For this review, take the finished solid that the model builds, in its own axes (mm). A direction names the side the tool comes from. Give positions to 0.01 mm unless a question says otherwise; leave off trailing zeros. Write each loop counter-clockwise with the first axis right and the second up, starting at its lowest first coordinate (ties: lowest second). Pieces come first, ordered by that corner, then holes. Notation, with made-up numbers: (57, -35) -> (106, -35) arc R21 cw to (106, -27) -> close; hole circle Ø2 at (41, -11.75). An arc over 180 degrees is marked (long way). Write item = value, one per line.
```python
from build123d import *

# Parameters (mm, degrees)
SKETCH1_R           = 28.4
BOSS_EXTRUDE1_DEPTH = 7
SKETCH2_R           = 28.4
BOSS_EXTRUDE3_DEPTH = 7
SKETCH4_R           = 7.5
BOSS_EXTRUDE4_DEPTH = 11
CUT_EXTRUDE1_DEPTH  = 10


with BuildPart() as part:
    # Sketch1 → Boss-Extrude1 (new body)
    with BuildSketch(Plane.XY):
        Circle(SKETCH1_R)
    extrude(amount=BOSS_EXTRUDE1_DEPTH)

    # Sketch2 → Boss-Extrude3 (add)
    with BuildSketch(Plane.XY.offset(7)):
        with Locations((1.88, 0)):
            Circle(SKETCH2_R)
    extrude(amount=BOSS_EXTRUDE3_DEPTH)

    # Sketch4 → Boss-Extrude4 (add)
    with BuildSketch(Plane.XY.offset(14)):
        with Locations((0.94, 0)):
            Circle(SKETCH4_R)
    extrude(amount=BOSS_EXTRUDE4_DEPTH)

    # Sketch6 → Cut-Extrude1 (cut)
    with BuildSketch(Plane.XY.offset(25)):
        with BuildLine():
            Line((0.44, 2.770056), (1.44, 2.770056))
            Line((1.44, 2.770056), (1.44, 4.472135955))
            ThreePointArc((1.44, 4.472135955), (0.94, -4.5), (0.44, 4.472135955))
            Line((0.44, 4.472135955), (0.44, 2.770056))
        make_face()
    extrude(amount=-CUT_EXTRUDE1_DEPTH, mode=Mode.SUBTRACT)


solid = part.part
```
(1) Tool access review of faces 1 (the face through (0.44, 4, 20)), 2 (the face through (-27, 2, 7)), 3 (the face through (29, 0, 7)): name each direction out of +Z, -Z, +X, -X, +Y, -Y from which nothing blocks a thin tool from reaching the whole face with its end or side.
Answers below:
face_1 = +Z
face_2 = +Z, -X
face_3 = -Z, +X
(2) Take a section at B-B (y = 0). Write out the cut boundary in (x, z).
Answers below:
outline = (-28.4, 0) -> (28.4, 0) -> (28.4, 7) -> (30.28, 7) -> (30.28, 14) -> (8.44, 14) -> (8.44, 25) -> (5.44, 25) -> (5.44, 15) -> (-3.56, 15) -> (-3.56, 25) -> (-6.56, 25) -> (-6.56, 14) -> (-26.52, 14) -> (-26.52, 7) -> (-28.4, 7) -> close
(3) To check wall thickness, follow probe 1 along Y at (x, z) = (0.94, 17); probe 2 along Z at (x, y) = (-17.5, -21); probe 3 along Z at (x, y) = (15, 20). State the ranges of each line that lie inside material, in increasing order.
Answers below:
probe_1 = -7.5 to -4.5, 2.77 to 7.5
probe_2 = 0 to 7
probe_3 = 0 to 14
(4) Take a section at D-D (z = 9.25). Write out the cut boundary in (x, y), plus the area to 3 significant figures.
Answers below:
outline = circle Ø56.8 at (1.88, 0)
area = 2,530 mm^2
(5) Take a section at A-A (z = 18). Write out the cut boundary in (x, y).
Answers below:
outline = circle Ø15 at (0.94, 0); hole (0.44, 2.77) -> (0.44, 4.47) arc R4.5 ccw (long way) to (1.44, 4.47) -> (1.44, 2.77) -> close
(6) For pin 1 (6 mm diameter, centred on x = -7.5, y = 9.5, fed in from +Z); pin 2 (1.4 mm diameter, centred on y = 4, z = 18, fed in from +X) (3 decimals); pin 3 (3 mm diameter, centred on x = -13.5, z = 4, fed in from -Y), all flat-tipped, find the tip position at first contact; note any pin that passes through.
Answers below:
pin_1 = 14
pin_2 = 7.675
pin_3 = -25.74
(7) Take a section at C-C (x = -5). Write out the cut boundary in (y, z), plus the area to 3 significant figures.
Answers below:
outline = (-27.96, 0) -> (27.96, 0) -> (27.96, 7) -> (27.55, 7) -> (27.55, 14) -> (4.58, 14) -> (4.58, 25) -> (-4.58, 25) -> (-4.58, 14) -> (-27.55, 14) -> (-27.55, 7) -> (-27.96, 7) -> close
area = 878 mm^2
